```python
from build123d import *

# Parameters (mm, degrees)
F0_R     = 14
F1_DEPTH = 30


with BuildPart() as f1:
    # F0 (on Top) → F1 (new body)
    with BuildSketch(Plane.XY):
        with BuildLine():
            Line((-23.6665773145, 17.4999972433), (-34.3713387844, 17.4999972433))
            ThreePointArc((-34.3713387844, 17.4999972433), (-36.3151814801, 16.0646276083), (-38.104839623, 14.4410715894))
            Line((-38.104839623, 14.4410715894), (-38.104839623, 5.9852786175))
            ThreePointArc((-38.104839623, 5.9852786175), (-37.2854541079, 7.4593001752), (-36.3385899052, 8.8548575392))
            ThreePointArc((-36.3385899052, 8.8548575392), (-36.4844121138, 12.8795697341), (-32.4596999189, 12.7337475255))
            ThreePointArc((-32.4596999189, 12.7337475255), (-28.3758248379, 15.053708361), (-23.8476290358, 16.3009840854))
            ThreePointArc((-23.8476290358, 16.3009840854), (-23.8240141463, 16.910594262), (-23.6665773145, 17.4999972433))
        make_face()
        with BuildLine():
            Line((-4.104839623, -10.985284131), (-4.104839623, 5.9852786175))
            ThreePointArc((-4.104839623, 5.9852786175), (-4.924225138, 7.4593001752), (-5.8710893408, 8.8548575392))
            ThreePointArc((-5.8710893408, 8.8548575392), (-9.6143544287, 8.9904824376), (-9.7499793271, 12.7337475255))
            ThreePointArc((-9.7499793271, 12.7337475255), (-13.833854408, 15.053708361), (-18.3620502102, 16.3009840854))
            ThreePointArc((-18.3620502102, 16.3009840854), (-21.104839623, 13.7499972433), (-23.8476290358, 16.3009840854))
            ThreePointArc((-23.8476290358, 16.3009840854), (-28.3758248379, 15.053708361), (-32.4596999189, 12.7337475255))
            ThreePointArc((-32.4596999189, 12.7337475255), (-31.9627612206, 11.8947230423), (-31.7898684655, 10.9350260858))
            ThreePointArc((-31.7898684655, 10.9350260858), (-33.3961866827, 8.4341278513), (-36.3385899052, 8.8548575392))
            ThreePointArc((-36.3385899052, 8.8548575392), (-37.2854541079, 7.4593001752), (-38.104839623, 5.9852786175))
            Line((-38.104839623, 5.9852786175), (-38.104839623, -10.985284131))
            ThreePointArc((-38.104839623, -10.985284131), (-37.2854541079, -12.4593056886), (-36.3385899052, -13.8548630526))
            ThreePointArc((-36.3385899052, -13.8548630526), (-33.3961866827, -13.4341333647), (-31.7898684655, -15.9350315993))
            ThreePointArc((-31.7898684655, -15.9350315993), (-31.9627612206, -16.8947285558), (-32.4596999189, -17.7337530389))
            ThreePointArc((-32.4596999189, -17.7337530389), (-28.3758248379, -20.0537138744), (-23.8476290358, -21.3009895988))
            ThreePointArc((-23.8476290358, -21.3009895988), (-21.104839623, -18.7500027567), (-18.3620502102, -21.3009895988))
            ThreePointArc((-18.3620502102, -21.3009895988), (-13.833854408, -20.0537138744), (-9.7499793271, -17.7337530389))
            ThreePointArc((-9.7499793271, -17.7337530389), (-9.6143544287, -13.990487951), (-5.8710893408, -13.8548630526))
            ThreePointArc((-5.8710893408, -13.8548630526), (-4.924225138, -12.4593056886), (-4.104839623, -10.985284131))
        make_face()
        with Locations((-21.104839623, -2.5000027567)):
            Circle(F0_R, mode=Mode.SUBTRACT)
        with BuildLine():
            Line((-4.104839623, 5.9852786175), (-4.104839623, 14.4410715894))
            ThreePointArc((-4.104839623, 14.4410715894), (-5.8944977658, 16.0646276083), (-7.8383404616, 17.4999972433))
            Line((-7.8383404616, 17.4999972433), (-18.5431019315, 17.4999972433))
            ThreePointArc((-18.5431019315, 17.4999972433), (-18.4023150022, 17.0087807672), (-18.354839623, 16.4999972433))
            ThreePointArc((-18.354839623, 16.4999972433), (-18.356642861, 16.4004253728), (-18.3620502102, 16.3009840854))
            ThreePointArc((-18.3620502102, 16.3009840854), (-13.833854408, 15.053708361), (-9.7499793271, 12.7337475255))
            ThreePointArc((-9.7499793271, 12.7337475255), (-6.7101138239, 13.5121333307), (-4.9198107804, 10.9350260858))
            ThreePointArc((-4.9198107804, 10.9350260858), (-5.1689125459, 9.791344303), (-5.8710893408, 8.8548575392))
            ThreePointArc((-5.8710893408, 8.8548575392), (-4.924225138, 7.4593001752), (-4.104839623, 5.9852786175))
        make_face()
        with BuildLine():
            ThreePointArc((-18.3620502102, 16.3009840854), (-21.104839623, 16.4999972433), (-23.8476290358, 16.3009840854))
            ThreePointArc((-23.8476290358, 16.3009840854), (-21.104839623, 13.7499972433), (-18.3620502102, 16.3009840854))
        make_face()
        with BuildLine():
            ThreePointArc((-18.354839623, 16.4999972433), (-18.4023150022, 17.0087807672), (-18.5431019315, 17.4999972433))
            Line((-18.5431019315, 17.4999972433), (-23.6665773145, 17.4999972433))
            ThreePointArc((-23.6665773145, 17.4999972433), (-23.8240141463, 16.910594262), (-23.8476290358, 16.3009840854))
            ThreePointArc((-23.8476290358, 16.3009840854), (-21.104839623, 16.4999972433), (-18.3620502102, 16.3009840854))
            ThreePointArc((-18.3620502102, 16.3009840854), (-18.356642861, 16.4004253728), (-18.354839623, 16.4999972433))
        make_face()
        with BuildLine():
            ThreePointArc((-18.3620502102, -21.3009895988), (-21.104839623, -18.7500027567), (-23.8476290358, -21.3009895988))
            ThreePointArc((-23.8476290358, -21.3009895988), (-21.104839623, -21.5000027567), (-18.3620502102, -21.3009895988))
        make_face()
        with BuildLine():
            ThreePointArc((-38.104839623, -19.4410771028), (-36.3151814801, -21.0646331217), (-34.3713387844, -22.5000027567))
            Line((-34.3713387844, -22.5000027567), (-23.6665773145, -22.5000027567))
            ThreePointArc((-23.6665773145, -22.5000027567), (-23.8240141463, -21.9105997754), (-23.8476290358, -21.3009895988))
            ThreePointArc((-23.8476290358, -21.3009895988), (-28.3758248379, -20.0537138744), (-32.4596999189, -17.7337530389))
            ThreePointArc((-32.4596999189, -17.7337530389), (-36.4844121138, -17.8795752475), (-36.3385899052, -13.8548630526))
            ThreePointArc((-36.3385899052, -13.8548630526), (-37.2854541079, -12.4593056886), (-38.104839623, -10.985284131))
            Line((-38.104839623, -10.985284131), (-38.104839623, -19.4410771028))
        make_face()
        with BuildLine():
            ThreePointArc((-7.8383404616, -22.5000027567), (-5.8944977658, -21.0646331217), (-4.104839623, -19.4410771028))
            Line((-4.104839623, -19.4410771028), (-4.104839623, -10.985284131))
            ThreePointArc((-4.104839623, -10.985284131), (-4.924225138, -12.4593056886), (-5.8710893408, -13.8548630526))
            ThreePointArc((-5.8710893408, -13.8548630526), (-5.1689125459, -14.7913498164), (-4.9198107804, -15.9350315993))
            ThreePointArc((-4.9198107804, -15.9350315993), (-6.7101138239, -18.5121388441), (-9.7499793271, -17.7337530389))
            ThreePointArc((-9.7499793271, -17.7337530389), (-13.833854408, -20.0537138744), (-18.3620502102, -21.3009895988))
            ThreePointArc((-18.3620502102, -21.3009895988), (-18.356642861, -21.4004308862), (-18.354839623, -21.5000027567))
            ThreePointArc((-18.354839623, -21.5000027567), (-18.4023150022, -22.0087862806), (-18.5431019315, -22.5000027567))
            Line((-18.5431019315, -22.5000027567), (-7.8383404616, -22.5000027567))
        make_face()
        with BuildLine():
            Line((-4.104839623, -22.5000027567), (-4.104839623, -19.4410771028))
            ThreePointArc((-4.104839623, -19.4410771028), (-5.8944977658, -21.0646331217), (-7.8383404616, -22.5000027567))
            Line((-7.8383404616, -22.5000027567), (-4.104839623, -22.5000027567))
        make_face()
        with BuildLine():
            Line((-38.104839623, -22.5000027567), (-34.3713387844, -22.5000027567))
            ThreePointArc((-34.3713387844, -22.5000027567), (-36.3151814801, -21.0646331217), (-38.104839623, -19.4410771028))
            Line((-38.104839623, -19.4410771028), (-38.104839623, -22.5000027567))
        make_face()
        with BuildLine():
            ThreePointArc((-38.104839623, 14.4410715894), (-36.3151814801, 16.0646276083), (-34.3713387844, 17.4999972433))
            Line((-34.3713387844, 17.4999972433), (-38.104839623, 17.4999972433))
            Line((-38.104839623, 17.4999972433), (-38.104839623, 14.4410715894))
        make_face()
        with BuildLine():
            ThreePointArc((-7.8383404616, 17.4999972433), (-5.8944977658, 16.0646276083), (-4.104839623, 14.4410715894))
            Line((-4.104839623, 14.4410715894), (-4.104839623, 17.4999972433))
            Line((-4.104839623, 17.4999972433), (-7.8383404616, 17.4999972433))
        make_face()
        with BuildLine():
            Line((-23.6665773145, -22.5000027567), (-18.5431019315, -22.5000027567))
            ThreePointArc((-18.5431019315, -22.5000027567), (-18.4023150022, -22.0087862806), (-18.354839623, -21.5000027567))
            ThreePointArc((-18.354839623, -21.5000027567), (-18.356642861, -21.4004308862), (-18.3620502102, -21.3009895988))
            ThreePointArc((-18.3620502102, -21.3009895988), (-21.104839623, -21.5000027567), (-23.8476290358, -21.3009895988))
            ThreePointArc((-23.8476290358, -21.3009895988), (-23.8240141463, -21.9105997754), (-23.6665773145, -22.5000027567))
        make_face()
    extrude(amount=F1_DEPTH)


solid = f1.part
```
Check sheet for the modelled part. Datum: model origin and axes. Units: mm. Round coordinates to 2 decimals unless told otherwise and drop trailing zeros. Order: outer loops, then holes, each group sorted by start corner. A loop starts at its lowest first (then second) coordinate and runs counter-clockwise, first axis right, second up.
1) Section check D-D (y = -14.5). Record the boundary of the cut face in (x, z).
2) Mould release check, pull along X, two halves, no side actions. Record for faces 1 (the flat face through (-38.105, -2, 15)), 2 (the flat face through (-4.105, -3, 15)), 3 (the flat face through (-21, -22.5, 15)), 4 (the cylindrical face through (-32.215, -11.019, 14.79)): +X half, -X half, draft (parallel to the pull), parting line (faces both ways), or undercut.
3) Section check C-C (y = -4.5). Record the boundary of the cut face in (x, z), and give its area (3 significant figures).
4) Scan lines: line 1 (X direction, y = -15, z = 28); line 2 (Y direction, x = -36, z = 19); line 3 (X direction, y = -14.5, z = 17.5). Record each from-to range of solid material in increasing order.
5) Section check A-A (z = 24.75). Record the boundary of the cut face in (x, y), and give its area (3 significant figures).
6) Section check B-B (x = -16.5). Record the boundary of the cut face in (y, z).
Result:
1. outline: (-38.1, 0) - (-36.89, 0) - (-36.89, 30) - (-38.1, 30) - close; (-32.19, 0) - (-28.32, 0) - (-28.32, 30) - (-32.19, 30) - close; (-13.89, 0) - (-10.02, 0) - (-10.02, 30) - (-13.89, 30) - close; (-5.32, 0) - (-4.1, 0) - (-4.1, 30) - (-5.32, 30) - close
2. face 1: -X half
2. face 2: +X half
2. face 3: draft
2. face 4: undercut
3. outline: (-38.1, 0) - (-34.96, 0) - (-34.96, 30) - (-38.1, 30) - close; (-7.25, 0) - (-4.1, 0) - (-4.1, 30) - (-7.25, 30) - close
3. area: 189 mm2
4. line 1: x = -38.1 to -37.13, -31.95 to -27.41, -14.8 to -10.26, -5.08 to -4.1
4. line 2: y = -22.5 to -18.27, -13.6 to 8.6, 13.27 to 17.5
4. line 3: x = -38.1 to -36.89, -32.19 to -28.32, -13.89 to -10.02, -5.32 to -4.1
5. outline: (-38.1, -22.5) - (-4.1, -22.5) - (-4.1, 17.5) - (-38.1, 17.5) - close; hole circle Ø5.5 at (-34.54, -15.94); hole circle Ø5.5 at (-34.54, 10.94); hole circle Ø28 at (-21.1, -2.5); hole circle Ø5.5 at (-7.67, -15.94); hole circle Ø5.5 at (-7.67, 10.94)
5. area: 649 mm2
6. outline: (-22.5, 0) - (-15.72, 0) - (-15.72, 30) - (-22.5, 30) - close; (10.72, 0) - (17.5, 0) - (17.5, 30) - (10.72, 30) - close
